Answer from the drawing. Dimensions are ordinates in mm from the lowest x, y and z of the part. Round coordinates to 2 decimals unless told otherwise and drop trailing zeros. Write each loop counter-clockwise with the first axis right and the second up, starting at its lowest first coordinate (ties: lowest second). Pieces come first, ordered by that corner, then holes. Notation, with made-up numbers: (4.25, 78) - (47.25, 78) arc R32 ccw to (47.25, 112) - close; hole circle Ø8 at (85, -0.75). An arc over 180 degrees is marked (long way). One line per item, written item: value. Start each with the question number.
(1) A cutting plane is placed at C-C, the plane z = 5. Determine the outline of the cut face in (x, y), plus the area to 3 significant figures.
(2) Find the intervals of material crossed by L1, parallel to X at y = 10, z = 1.5; L2, parallel to Y at x = 41, z = 0.3; L3, parallel to Y at x = 7.5, z = 2.2, in increasing order.
(3) A flat-ended cylindrical pin translates along its axis: pin 1 Ø5.5 at (x, y) = (9, 10) entering from +Z. Find the tip coordinate at first contact, or state that the pin passes through.
(4) A cutting plane is placed at B-B, the plane x = 9. Determine the outline of the cut face in (y, z), plus the area to 3 significant figures.
(5) A cutting plane is placed at A-A, the plane y = 20. Determine the outline of the cut face in (x, z), plus the area to 3 significant figures.
(6) The mould has two halves that part along Y. Classify the marked faces 1, 2, 3 and 4: +Y half, -Y half, draft (parallel to the pull), parting line (faces both ways), or undercut.
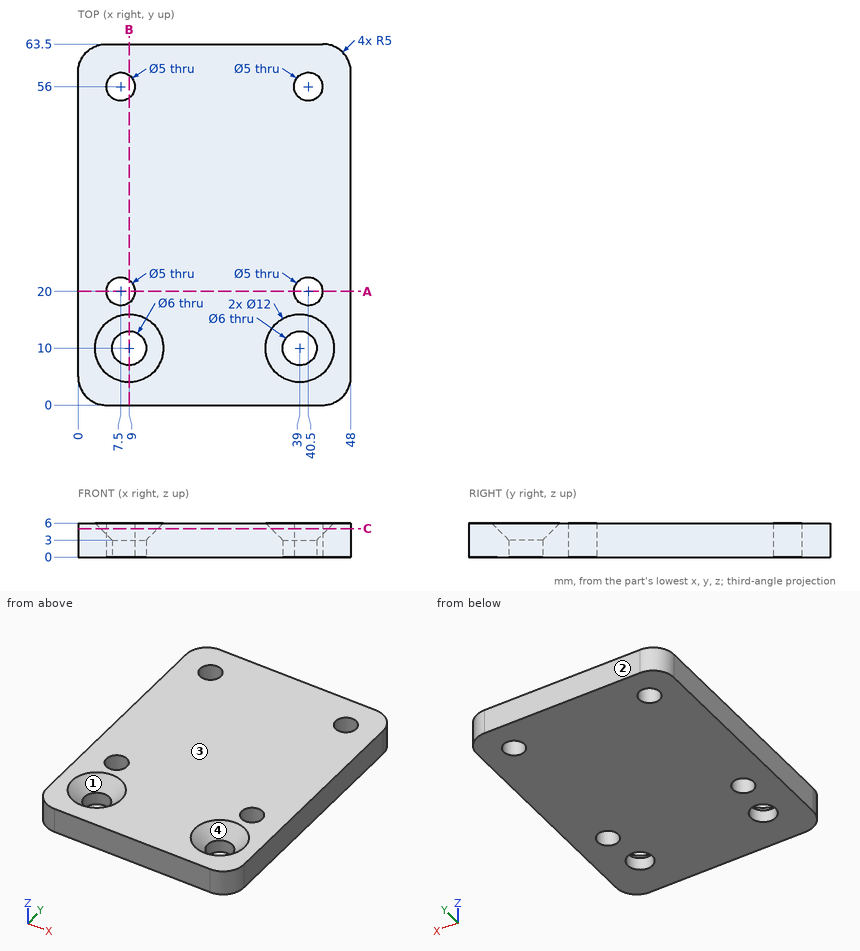
Here are the results:
1. outline: (0, 5) arc R5 ccw to (5, 0) - (43, 0) arc R5 ccw to (48, 5) - (48, 58.5) arc R5 ccw to (43, 63.5) - (5, 63.5) arc R5 ccw to (0, 58.5) - close; hole circle Ø10 at (9, 10); hole circle Ø5 at (7.5, 20); hole circle Ø5 at (7.5, 56); hole circle Ø10 at (39, 10); hole circle Ø5 at (40.5, 20); hole circle Ø5 at (40.5, 56)
1. area: 2,790 mm²
2. L1: 0 to 6, 12 to 36, 42 to 48
2. L2: 0 to 7.76, 12.24 to 17.55, 22.45 to 53.55, 58.45 to 63.5
2. L3: 0 to 7.4, 12.6 to 17.5, 22.5 to 53.5, 58.5 to 63.5
3. pin 1: through
4. outline: (0, 0) - (7, 0) - (7, 3) - (4, 6) - (0, 6) - close; (13, 0) - (18, 0) - (18, 6) - (16, 6) - (13, 3) - close; (22, 0) - (54, 0) - (54, 6) - (22, 6) - close; (58, 0) - (63.5, 0) - (63.5, 6) - (58, 6) - close
4. area: 288 mm²
5. outline: (0, 0) - (5, 0) - (5, 6) - (0, 6) - close; (10, 0) - (38, 0) - (38, 6) - (10, 6) - close; (43, 0) - (48, 0) - (48, 6) - (43, 6) - close
5. area: 228 mm²
6. face 1: undercut
6. face 2: +Y half
6. face 3: draft
6. face 4: undercut
